from build123d import *

# Parameters (mm, degrees)
CROQUIS1_W              = 20
CROQUIS1_H              = 100
SALIENTE_EXTRUIR1_DEPTH = 240
CROQUIS2_W              = 19
CROQUIS2_H              = 9
CORTAR_EXTRUIR1_DEPTH   = 240
CROQUIS3_R              = 2
CROQUIS3_W              = 238
CROQUIS3_H              = 90
CORTAR_EXTRUIR2_DEPTH   = 19
CROQUIS4_W              = 1
CROQUIS4_H              = 90
CORTAR_EXTRUIR3_DEPTH   = 9
CROQUIS5_R              = 7.5
CROQUIS5_W              = 240
CROQUIS5_H              = 10
CORTAR_EXTRUIR5_DEPTH   = 20


with BuildPart() as part:
    # Croquis1 → Saliente-Extruir1 (new body)
    with BuildSketch(Plane.XY):
        with Locations((7.330646947, -26.197398527)):
            Rectangle(CROQUIS1_W, CROQUIS1_H)
    extrude(amount=SALIENTE_EXTRUIR1_DEPTH)

    # Croquis2 → Cortar-Extruir1 (cut)
    with BuildSketch(Plane.XY.offset(240)):
        with Locations((7.830646947, 19.302601473)):
            Rectangle(CROQUIS2_W, CROQUIS2_H)
    extrude(amount=-CORTAR_EXTRUIR1_DEPTH, mode=Mode.SUBTRACT)

    # Croquis3 → Cortar-Extruir2 (cut)
    with BuildSketch(Plane.ZY.offset(2.669353053)):
        with Locations((40, 19.302601473)):
            Circle(CROQUIS3_R)
        with Locations((200, 19.302601473)):
            Circle(CROQUIS3_R)
        with Locations((120, -31.197398527)):
            Rectangle(CROQUIS3_W, CROQUIS3_H)
    extrude(amount=-CORTAR_EXTRUIR2_DEPTH, mode=Mode.SUBTRACT)

    # Croquis4 → Cortar-Extruir3 (cut)
    with BuildSketch(Plane.ZY.offset(2.669353053)):
        with Locations((0.5, -31.197398527)):
            Rectangle(CROQUIS4_W, CROQUIS4_H)
        with Locations((239.5, -31.197398527)):
            Rectangle(CROQUIS4_W, CROQUIS4_H)
    extrude(amount=-CORTAR_EXTRUIR3_DEPTH, mode=Mode.SUBTRACT)

    # Croquis5 → Cortar-Extruir5 (cut)
    with BuildSketch(Plane(origin=(17.330646947, 0, 0), x_dir=(0, 0, -1), z_dir=(1, 0, 0))):
        with Locations((-200, -30.197398527)):
            Circle(CROQUIS5_R)
        with Locations((-40, -30.197398527)):
            Circle(CROQUIS5_R)
        with Locations((-120, -71.197398527)):
            Rectangle(CROQUIS5_W, CROQUIS5_H)
    extrude(amount=-CORTAR_EXTRUIR5_DEPTH, mode=Mode.SUBTRACT)


solid = part.part
The model under review builds one solid part; all positions refer to its coordinate system, in mm. A direction names the side the tool comes from. Give positions to 0.01 mm unless a question says otherwise; leave off trailing zeros. Order: outer loops, then holes, each group sorted by start corner. A loop starts at its lowest first (then second) coordinate and runs counter-clockwise, first axis right, second up. Notation, with made-up numbers: (59, 72.5) -> (88, 72.5) arc R13 cw to (88, 95.5) -> close; hole circle Ø7 at (42, -15). An arc over 180 degrees is marked (long way). Write item = value, one per line. Start each with the question number.
(1) For pin 1 Ø5.5 at (x, z) = (10.5, 116) entering from +Y; pin 2 Ø1.1 at (y, z) = (-34, 239.5) entering from -X; pin 3 Ø6 at (x, z) = (11, 185) entering from -Y; pin 4 Ø12 at (y, z) = (-30.2, 40) entering from -X, all flat-tipped, find the tip position at first contact; note any pin that passes through.
(2) Tool access review of faces 5 (the flat face through (8, 14.803, 122)), 6 (the cylindrical face through (16.84, -23.87, 35.97)), 7 (the flat face through (11, -27, 239)): name each direction out of +Z, -Z, +X, -X, +Y, -Y from which nothing blocks a thin tool from reaching the whole face with its end or side.
(3) Take a section at A-A (y = 3). Write out the cut boundary in (x, z).
(4) For L1, parallel to Y at x = 16.6, z = 40; L2, parallel to Z at x = 7.25, y = -17; L3, parallel to Y at x = -2, z = 200, list the stretches that pass through material, from the lowest coordinate up. Write a range as from..to.
(5) Take a section at B-B (z = 220). Write out the cut boundary in (x, y), plus the area to 3 significant figures.
(6) Draft analysis for pull direction Z (two halves, no side actions). For faces 1 (the flat face through (-1.669, 19, 122)), 2 (the flat face through (12, -21, 240)), 3 (the flat face through (16.331, -26, 118)), 4 (the cylindrical face through (-2.18, 19.39, 198)), state which applies: +Z half, -Z half, draft (parallel to the pull), parting line (faces both ways), or undercut.
Returned:
q1.pin_1 = 14.8
q1.pin_2 = 6.33
q1.pin_3 = 13.8
q1.pin_4 = through
q2.face_5 = +Z, -Z, +X, +Y
q2.face_6 = +X, -X
q2.face_7 = -X, -Y
q3.outline = (6.33, 0) -> (17.33, 0) -> (17.33, 240) -> (6.33, 240) -> (6.33, 239) -> (16.33, 239) -> (16.33, 1) -> (6.33, 1) -> close
q4.L1 = -66.2..-37.7, -22.7..14.8
q4.L2 = 0..1, 239..240
q4.L3 = 13.8..17.3, 21.3..23.8
q5.outline = (-2.67, 13.8) -> (16.33, 13.8) -> (16.33, -66.2) -> (17.33, -66.2) -> (17.33, 14.8) -> (-1.67, 14.8) -> (-1.67, 23.8) -> (-2.67, 23.8) -> close
q5.area = 109 mm²
q6.face_1 = draft
q6.face_2 = +Z half
q6.face_3 = undercut
q6.face_4 = undercut
